Input: part model. Units: mm. Frame: model coordinates. Give positions to 0.01 mm unless a question says otherwise; leave off trailing zeros. Loops run counter-clockwise (first coordinate to the right, second up) from the corner with the lowest first, then second, coordinate; pieces in that order, holes last. Notation, with made-up numbers: (-24, 61.25) -> (20, 61.25) arc R33 cw to (20, 91.25) -> close; hole circle Ø1 at (33, 49.5). An arc over 180 degrees is marked (long way). One line per question, with ' | ' between items.
from build123d import *

# Parameters (mm, degrees)
F1_DEPTH = 50
F2_SIZE  = 49.99999
F3_DEPTH = 20


# Not quite as in the source:
# - a fillet or chamfer is up to 0.001 mm smaller than in the source, because OpenCascade refuses the exact size


with BuildPart() as f1:
    # F0 (on Front) → F1 (new body)
    with BuildSketch(Plane.XZ):
        Polygon((291.8585808619, -291.8585808619), (412.7503633499, 0), (291.8585808619, 291.8585808619), (0, 412.7503633499), (-291.8585808619, 291.8585808619), (-412.7503633499, 0), (-291.8585808619, -291.8585808619), (0, -412.7503633499), align=None)
    extrude(amount=F1_DEPTH)

    # F2 (size 50 in the source; OpenCascade refuses exactly that, so slightly less here)
    f2_edges = [f1.edges().sort_by_distance(p)[0] for p in [
        (-352.304472, -50, -145.92929),
        (-145.92929, -50, -352.304472),
        (145.92929, -50, -352.304472),
        (352.304472, -50, -145.92929),
        (352.304472, -50, 145.92929),
        (145.92929, -50, 352.304472),
        (-145.92929, -50, 352.304472),
        (-352.304472, -50, 145.92929),
    ]]
    chamfer(f2_edges, length=F2_SIZE)

    # F0 (on Front) → F3 (join)
    with BuildSketch(Plane.XZ):
        Polygon((291.8585808619, -291.8585808619), (412.7503633499, 0), (291.8585808619, 291.8585808619), (0, 412.7503633499), (-291.8585808619, 291.8585808619), (-412.7503633499, 0), (-291.8585808619, -291.8585808619), (0, -412.7503633499), align=None)
    extrude(amount=-F3_DEPTH)


solid = f1.part
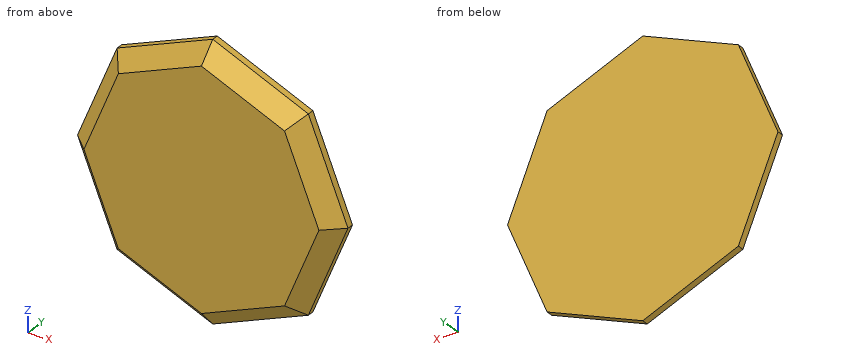
1. Ray query, line 1 along Z through (x, y) = (209.5, 3.5); line 2 along Z through (x, y) = (-366, 2); line 3 along X through (y, z) = (-28, -229). Return the intervals inside material, ascending. Write a range as from..to.
Determined:
line 1: z = -325.97..325.97 | line 2: z = -112.87..112.87 | line 3: x = -287.59..287.59
2. Pin query (flat end, axial travel): P1, Ø1, axis at y = -10.5, z = 108.5, coming from the -X side; P2, Ø6, axis at y = -39.5, z = 171, coming from the -X side; P3, Ø2, axis at x = 53, y = -17.5, coming from the -Z side. Return the tip coordinate at first contact, or that it passes through.
Determined:
P1: stops at x = -357.02 | P2: stops at x = -302.64 | P3: stops at z = -373.01
3. Section query B-B (x = 127.5). Output: boundary loops of the cut face in (y, z), then the cut area to 3 significant figures.
Determined:
outline: (-50, -305.82) -> (0, -359.94) -> (20, -359.94) -> (20, 359.94) -> (0, 359.94) -> (-50, 305.82) -> close | area: 47,700 mm2
4. Section query C-C (z = -302). Output: boundary loops of the cut face in (x, y), then the cut area to 3 significant figures.
Determined:
outline: (-267.38, 0) -> (-136.72, -50) -> (136.72, -50) -> (267.38, 0) -> (267.38, 20) -> (-267.38, 20) -> close | area: 30,900 mm2
5. Section query A-A (y = -17). Output: boundary loops of the cut face in (x, z).
Determined:
outline: (-394.35, 0) -> (-278.85, -278.85) -> (0, -394.35) -> (278.85, -278.85) -> (394.35, 0) -> (278.85, 278.85) -> (0, 394.35) -> (-278.85, 278.85) -> close
